Design review of the part built by this model. Coordinates are the model's own, in mm. Coordinates: 2 decimals unless noted, no trailing zeros. Loops run counter-clockwise (first coordinate to the right, second up) from the corner with the lowest first, then second, coordinate; pieces in that order, holes last.
Q1. Add section B-B on z = 2.5. Give the boundary of the cut face in (x, y).
Q2. Add section A-A on x = 14.25. Give the boundary of the cut face in (y, z).
Q3. Wall thickness on probe 1 along X at (y, z) = (1.25, 8); probe 2 along Z at (x, y) = (16, 3); probe 3 along X at (y, z) = (3.5, 13.5): over which ranges is each line inside the solid? List them lowest first.
Q4. For P1, Ø10, axis at x = 17, y = 8, coming from the +Z side; P2, Ø3, axis at y = 4, z = 12.5, coming from the +X side; P3, Ø1.5, axis at x = 17, y = 5, coming from the -Z side; P4, Ø1.5, axis at x = 13.5, y = 2, coming from the +Z side, all flat-tipped, find the tip position at first contact; note any pin that passes through.
```python
from build123d import *

# Parameters (mm, degrees)
SKETCH1_W           = 20
SKETCH1_H           = 20
BOSS_EXTRUDE1_DEPTH = 20
CUT_EXTRUDE1_DEPTH  = 20
CUT_EXTRUDE2_DEPTH  = 20


with BuildPart() as part:
    # Sketch1 → Boss-Extrude1 (new body)
    with BuildSketch(Plane.XY):
        with Locations((10, 10)):
            Rectangle(SKETCH1_W, SKETCH1_H)
    extrude(amount=BOSS_EXTRUDE1_DEPTH)

    # Sketch2 → Cut-Extrude1 (cut)
    with BuildSketch(Plane(origin=(0, 20, 0), x_dir=(1, 0, 0), z_dir=(0, 1, 0))):
        Polygon((0, 0), (10, -20), (0, -20), align=None)
    extrude(amount=-CUT_EXTRUDE1_DEPTH, mode=Mode.SUBTRACT)

    # Sketch3 → Cut-Extrude2 (cut)
    with BuildSketch(Plane(origin=(0, 20, 0), x_dir=(1, 0, 0), z_dir=(0, 1, 0))):
        Polygon((20, -20), (20, -10), (10, -20), align=None)
    extrude(amount=-CUT_EXTRUDE2_DEPTH, mode=Mode.SUBTRACT)


solid = part.part
```
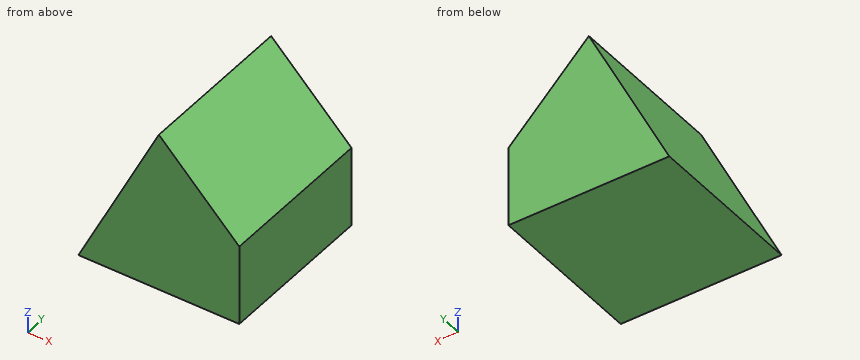
Entries:
1. outline: (1.25, 0) - (20, 0) - (20, 20) - (1.25, 20) - close
2. outline: (0, 0) - (20, 0) - (20, 15.75) - (0, 15.75) - close
3. probe 1: x = 4 to 20
3. probe 2: z = 0 to 14
3. probe 3: x = 6.75 to 16.5
4. P1: stops at z = 18
4. P2: stops at x = 19
4. P3: stops at z = 0
4. P4: stops at z = 17.25
